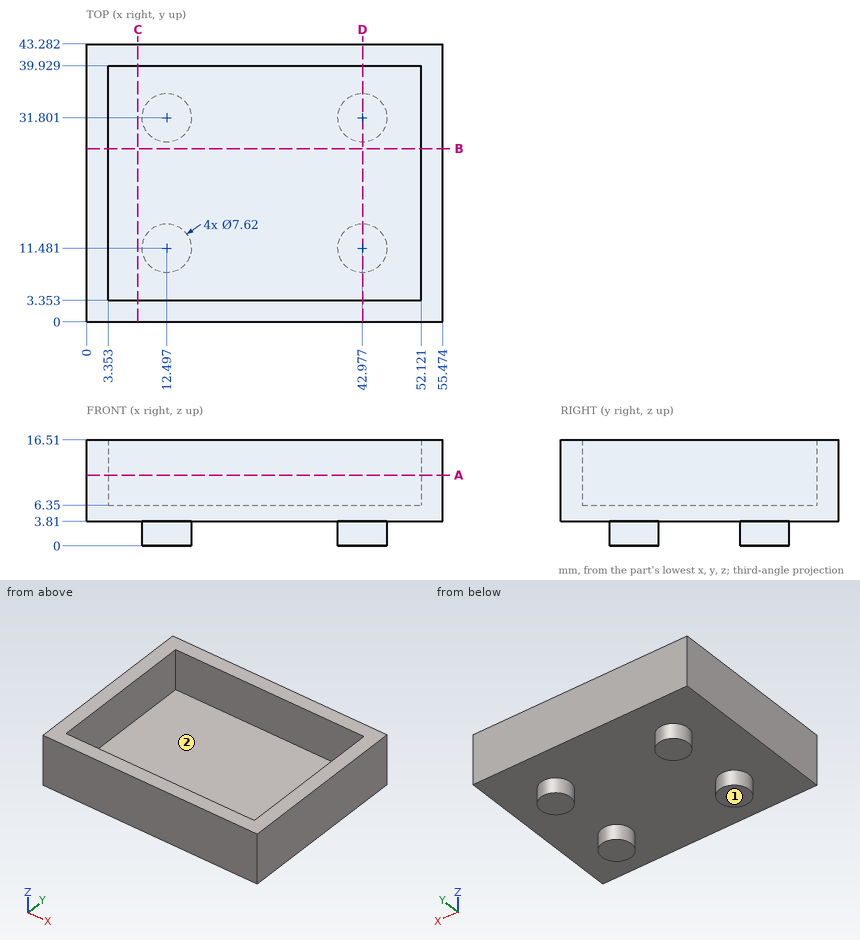
Job drawing, mm, ordinate dimensions from the low corner. One solid piece. A direction names the side the tool comes from. Round coordinates to 2 decimals unless told otherwise and drop trailing zeros. Order: outer loops, then holes, each group sorted by start corner. A loop starts at its lowest first (then second) coordinate and runs counter-clockwise, first axis right, second up. Notation, with made-up numbers: M 43,50.25 L 72,50.25 A28 ccw 72,80.25 Z; hole C 14.5,-26.75 d1. An arc over 180 degrees is marked long. Write each question's results on one line, items separated by ' | '. Start each with the question number.
(1) Which spindle directions (+Z, -Z, +X, -X, +Y, -Y) get a long thin tool onto all of the face, cutting with end or side? Do the marked faces 1 and 2. Say none if no direction does.
(2) Saw through at B-B, the plane y = 27. Give the cut face in (x, z), then the cut area to 3 significant figures.
(3) Probe probe 1 along Y at (x, z) = (45, 11.75); probe 2 along X at (y, z) = (7.5, 11.25); probe 3 along Z at (x, y) = (43, 12). List the from-to ranges inside material, lowest first. Write a range as from..to.
(4) Drop flat-ended pins along their axis: pin 1 (5 mm diameter, centred on x = 25.5, y = 21, fed in from +Z); pin 2 (6 mm diameter, centred on x = 28.5, y = 16, fed in from -Z). Give the stop position or say it passes through.
(5) Saw through at D-D, the plane x = 43. Give the cut face in (y, z).
(6) Saw through at C-C, the plane x = 8. Give the cut face in (y, z).
(7) Saw through at A-A, the plane z = 11. Give the cut face in (x, y).
Established:
1) face 1: -Z, +X, -X, +Y, -Y | face 2: +Z
2) outline: M 0,3.81 L 55.47,3.81 L 55.47,16.51 L 52.12,16.51 L 52.12,6.35 L 3.35,6.35 L 3.35,16.51 L 0,16.51 Z | area: 209 mm^2
3) probe 1: y = 0..3.35, 39.93..43.28 | probe 2: x = 0..3.35, 52.12..55.47 | probe 3: z = 0..6.35
4) pin 1: stops at z = 6.35 | pin 2: stops at z = 3.81
5) outline: M 0,3.81 L 7.67,3.81 L 7.67,0 L 15.29,0 L 15.29,3.81 L 27.99,3.81 L 27.99,0 L 35.61,0 L 35.61,3.81 L 43.28,3.81 L 43.28,16.51 L 39.93,16.51 L 39.93,6.35 L 3.35,6.35 L 3.35,16.51 L 0,16.51 Z
6) outline: M 0,3.81 L 43.28,3.81 L 43.28,16.51 L 39.93,16.51 L 39.93,6.35 L 3.35,6.35 L 3.35,16.51 L 0,16.51 Z
7) outline: M 0,0 L 55.47,0 L 55.47,43.28 L 0,43.28 Z; hole M 3.35,3.35 L 52.12,3.35 L 52.12,39.93 L 3.35,39.93 Z
